Verification items for this drawing (mm, ordinates from the low corner). Coordinates: 2 decimals unless noted, no trailing zeros. Order: outer loops, then holes, each group sorted by start corner. A loop starts at its lowest first (then second) coordinate and runs counter-clockwise, first axis right, second up. Notation, with made-up numbers: M 84,81 L 136,81 A14 cw 136,95 Z; hole C 33,-36.5 d3. An arc over 180 degrees is marked long. Write item = value, one per line.
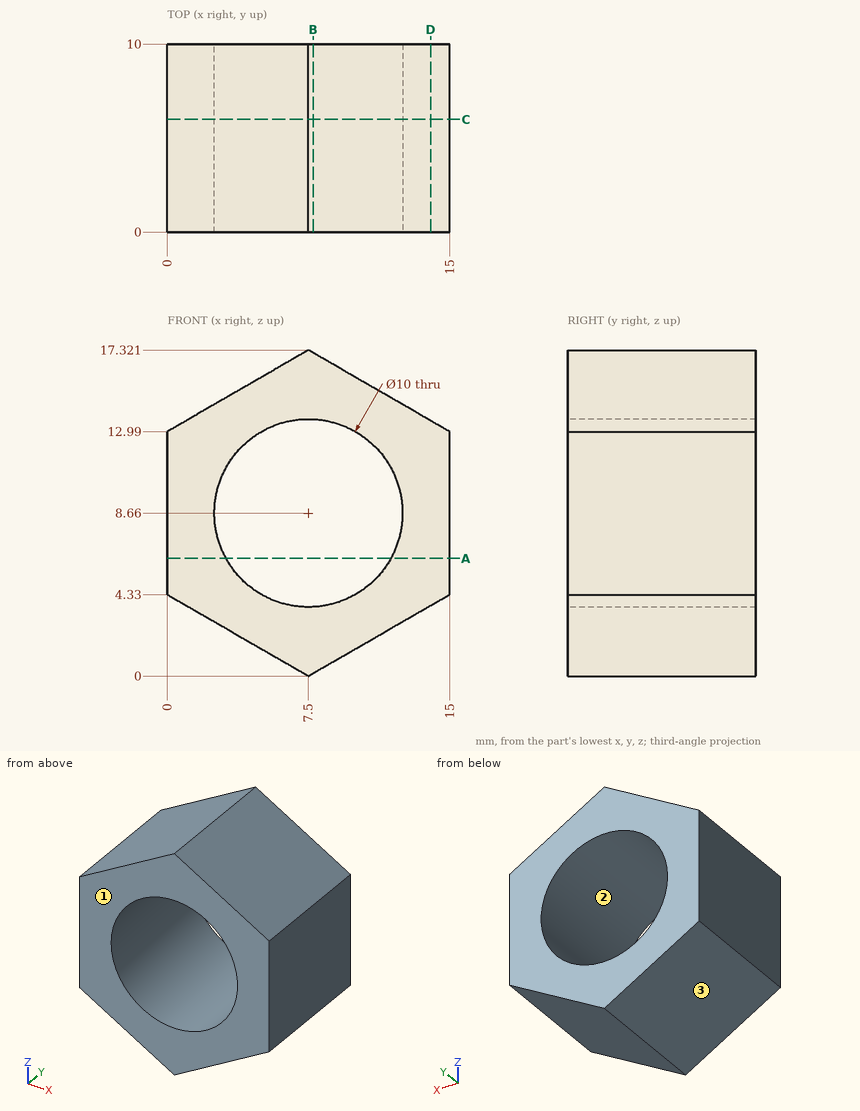
Item 1: Sectioned sample at B-B, the plane x = 7.75. Enter the section's corners in (y, z) (1 decimal).
Report:
outline = M 0,0.1 L 10,0.1 L 10,3.7 L 0,3.7 Z; M 0,13.7 L 10,13.7 L 10,17.2 L 0,17.2 Z
Item 2: Sectioned sample at A-A, the plane z = 6.25. Enter the section's corners in (x, y).
Report:
outline = M 0,0 L 3.12,0 L 3.12,10 L 0,10 Z; M 11.88,0 L 15,0 L 15,10 L 11.88,10 Z
Item 3: Scan lines: L1, parallel to X at y = 3.5, z = 12.5 (1 decimal); L2, parallel to Z at x = 5.5, y = 8 (1 decimal); L3, parallel to Z at x = 5.25, y = 8.75 (1 decimal). Record each from-to range of solid material in increasing order. Write a range as from..to.
Report:
L1 = 0..4.3, 10.7..15
L2 = 1.2..4.1, 13.2..16.2
L3 = 1.3..4.2, 13.1..16
Item 4: Gauge pin test, flat ends, axial feed: pin 1 (4 mm diameter, centred on x = 13.5, y = 6.5, fed in from -Z); pin 2 (6 mm diameter, centred on x = 7.5, z = 8.66, fed in from -Y); pin 3 (1.5 mm diameter, centred on y = 4, z = 14, fed in from -X). Record the tip position at first contact, or that the pin passes through.
Report:
pin_1 = 2.31
pin_2 = through
pin_3 = 0.45
Item 5: Sectioned sample at D-D, the plane x = 14. Enter the section's corners in (y, z).
Report:
outline = M 0,3.75 L 10,3.75 L 10,13.57 L 0,13.57 Z
Item 6: Release check for a two-part mould opening along Z. For the marked faces 1, 2 and 3 record: pulls with the +Z half, pulls with the -Z half, needs draft (parallel to the pull), parting line crosses it, or undercut.
Report:
face_1 = needs draft
face_2 = undercut
face_3 = pulls with the -Z half
Item 7: Sectioned sample at C-C, the plane y = 6. Enter the section's corners in (x, z).
Report:
outline = M 0,4.33 L 7.5,0 L 15,4.33 L 15,12.99 L 7.5,17.32 L 0,12.99 Z; hole C 7.5,8.66 d10
